Can you work these out from the model? Positions are in its coordinate system, mm. A direction names the side the tool comes from. Give positions to 0.01 mm unless a question says otherwise; leave off trailing zeros. Loops run counter-clockwise (first coordinate to the right, second up) from the corner with the lowest first, then second, coordinate; pieces in that order, holes last. Notation, with made-up numbers: M 25,-38 L 74,-38 A32 cw 74,-11 Z; hole C -32,11 d5. An arc over 180 degrees is marked long. Put each result on its own line as item: value. Start each with the question number.
1) For faces 4 (the cylindrical face through (6.14, 5.07, -21.94)), 5 (the flat face through (40, 5, -11)), 6 (the cylindrical face through (0.285, 5.07, -4.203)), which set-ups out of +Z, -Z, +X, -X, +Y, -Y let a thin tool reach every point of the face, with its end or its side?
2) Imagine slicing it at A-A (x = 16.5). Write out the boundary of the cut face in (y, z), then the cut area to 3 significant figures.
3) Imagine slicing it at C-C (z = -8.5). Write out the boundary of the cut face in (x, y).
4) Imagine slicing it at D-D (z = -31.5). Write out the boundary of the cut face in (x, y).
5) Please list where these lines run through material, in increasing order: line 1 along Z through (x, y) = (15, 4.75); line 2 along Z through (x, y) = (4.5, 7.75); line 3 along X through (y, z) = (9.25, -34.5). Write a range as from..to.
6) For P1, Ø3, axis at x = 30.5, z = -22.5, coming from the +Y side, with a flat end and sliding along its axis, tell me the tip position at first contact or that it passes through.
7) If we mould it in two halves opening along Z, with no side actions, what happens to faces 1 (the flat face through (20, 10, -20)), 2 (the cylindrical face through (38.797, 5.07, -1.141)), 3 (the cylindrical face through (38.859, 5.07, -20.455))? For each: +Z half, -Z half, draft (parallel to the pull), parting line (faces both ways), or undercut.
8) Imagine slicing it at B-B (y = 8). Write out the boundary of the cut face in (x, z), then the cut area to 3 significant figures.
from build123d import *

# Parameters (mm, degrees)
BOSS_EXTRUDE1_DEPTH = 10
FILLET1_R           = 4
FILLET2_R           = 1


with BuildPart() as part:
    # Sketch1 → Boss-Extrude1 (new body)
    with BuildSketch(Plane(origin=(0, 0, 0), x_dir=(1, 0, 0), z_dir=(0, 1, 0))):
        Polygon((0, 4.504109696), (0, 0), (33.415268294, 0), (40, 0), (40, 4.504109696), (40, 18.518496951), (40, 21.657719696), (33.415268294, 21.657719696), (5.834954176, 21.657719696), (5.834954176, 35.784222049), (40, 35.784222049), (40, 40), (5.834954176, 40), (0, 40), (0, 35.784222049), (0, 21.657719696), (0, 18.518496951), (33.415268294, 18.518496951), (33.415268294, 4.504109696), align=None)
    extrude(amount=BOSS_EXTRUDE1_DEPTH)

    # Fillet1
    fillet1_edges = [part.edges().sort_by_distance(p)[0] for p in [
        (0, 5, -18.518496951),
        (0, 5, -40),
        (40, 5, -21.657719696),
        (40, 5, 0),
    ]]
    fillet(fillet1_edges, radius=FILLET1_R)

    # Fillet2
    fillet2_edges = [part.edges().sort_by_distance(p)[0] for p in [
        (33.415268294, 5, -18.518496951),
        (40, 5, -40),
        (40, 5, -35.784222049),
        (5.834954176, 5, -35.784222049),
        (5.834954176, 5, -21.657719696),
        (0, 5, 0),
        (0, 5, -4.504109696),
        (33.415268294, 5, -4.504109696),
    ]]
    fillet(fillet2_edges, radius=FILLET2_R)


solid = part.part
Recorded:
1. face 4: +X, +Y, -Y
1. face 5: +Z, -Z, +X, +Y, -Y
1. face 6: -X, +Y, -Y
2. outline: M 0,-40 L 10,-40 L 10,-35.78 L 0,-35.78 Z; M 0,-21.66 L 10,-21.66 L 10,-18.52 L 0,-18.52 Z; M 0,-4.5 L 10,-4.5 L 10,0 L 0,0 Z
2. area: 119 mm²
3. outline: M 33.42,0 L 40,0 L 40,10 L 33.42,10 Z
4. outline: M 0,0 L 5.83,0 L 5.83,10 L 0,10 Z
5. line 1: -40..-35.78, -21.66..-18.52, -4.5..0
5. line 2: -40..-18.52, -4.5..0
5. line 3: 0..5.83
6. P1: y = 10
7. face 1: draft
7. face 2: +Z half
7. face 3: undercut
8. outline: M 0,-36 A4 ccw 4,-40 L 39,-40 A1 ccw 40,-39 L 40,-36.78 A1 ccw 39,-35.78 L 6.83,-35.78 A1 cw 5.83,-34.78 L 5.83,-22.66 A1 cw 6.83,-21.66 L 36,-21.66 A4 ccw 40,-17.66 L 40,-4 A4 ccw 36,0 L 1,0 A1 ccw 0,-1 L 0,-3.5 A1 ccw 1,-4.5 L 32.42,-4.5 A1 cw 33.42,-5.5 L 33.42,-17.52 A1 cw 32.42,-18.52 L 4,-18.52 A4 ccw 0,-22.52 Z
8. area: 635 mm²
